Part model, mm, in its own coordinate system. A direction names the side the tool comes from. Round coordinates to 2 decimals unless told otherwise and drop trailing zeros. Loops run counter-clockwise (first coordinate to the right, second up) from the corner with the lowest first, then second, coordinate; pieces in that order, holes last. Notation, with made-up numbers: M -15,-7.5 L 0,-7.5 A16 ccw 0,8.5 Z; hole C 17,87 d9. An arc over 180 degrees is marked long. Write each question's results on one line, items separated by ' | '.
from build123d import *

# Parameters (mm, degrees)
SKETCH_W      = 13
SKETCH_H      = 10
PAD_DEPTH     = 1.6
SKETCH001_R   = 1.5
SKETCH001_W   = 0.65
SKETCH001_H   = 0.65
POCKET_DEPTH  = 5
SKETCH002_W   = 2.6
SKETCH002_H   = 2.6
PAD001_DEPTH  = 0.03
SKETCH003_W   = 2.1
SKETCH003_H   = 2.1
PAD002_DEPTH  = 0.9
FILLET_R      = 0.3
FILLET001_R   = 0.05
FILLET002_R   = 0.2
SKETCH004_W   = 1.1
SKETCH004_H   = 2
SKETCH004_W_2 = 1.5
SKETCH004_H_2 = 0.9
SKETCH004_H_3 = 0.75
SKETCH004_H_4 = 2.9
SKETCH004_W_3 = 3.2
SKETCH004_H_5 = 1.4
SKETCH004_W_4 = 0.8
SKETCH004_H_6 = 1.6
PAD003_DEPTH  = 0.27
SKETCH005_W   = 2.4
SKETCH005_H   = 2.4
PAD004_DEPTH  = 2.4
CHAMFER_SIZE  = 0.5
PAD005_DEPTH  = 2.4
SKETCH007_W   = 0.65
SKETCH007_H   = 0.65
PAD006_DEPTH  = 12


with BuildPart() as part:
    # Sketch (on XY_Plane of Origin) → Pad (new body)
    with BuildSketch(Plane.XY):
        with Locations((6.5, 5)):
            Rectangle(SKETCH_W, SKETCH_H)
    extrude(amount=PAD_DEPTH)

    # Sketch001 (on XY_Plane of Origin) → Pocket (cut)
    with BuildSketch(Plane.XY):
        with Locations((10.4, 7.6)):
            Circle(SKETCH001_R)
        with Locations((1.4, 8.6)):
            Rectangle(SKETCH001_W, SKETCH001_H)
        with Locations((1.4, 6.2)):
            Rectangle(SKETCH001_W, SKETCH001_H)
        with Locations((1.4, 3.8)):
            Rectangle(SKETCH001_W, SKETCH001_H)
        with Locations((1.4, 1.4)):
            Rectangle(SKETCH001_W, SKETCH001_H)
    extrude(amount=POCKET_DEPTH, mode=Mode.SUBTRACT)

    # Sketch002 (on Face5 of Pocket) → Pad001 (join)
    with BuildSketch(Plane.XY.offset(1.6)):
        with Locations((10.6, 2.7)):
            Rectangle(SKETCH002_W, SKETCH002_H)
    extrude(amount=PAD001_DEPTH)

    # Sketch003 (on Face28 of Pad001) → Pad002 (join)
    with BuildSketch(Plane.XY.offset(1.63)):
        with Locations((10.6, 2.7)):
            Rectangle(SKETCH003_W, SKETCH003_H)
    extrude(amount=PAD002_DEPTH)

    # Fillet
    fillet_edges = [part.edges().sort_by_distance(p)[0] for p in [
        (9.55, 1.65, 2.08),
        (9.55, 3.75, 2.08),
        (11.65, 1.65, 2.08),
        (11.65, 3.75, 2.08),
    ]]
    fillet(fillet_edges, radius=FILLET_R)

    # Fillet001
    fillet001_edges = [part.edges().sort_by_distance(p)[0] for p in [
        (9.637868, 1.737868, 1.63),
    ]]
    fillet(fillet001_edges, radius=FILLET001_R)

    # Fillet002
    fillet002_edges = [part.edges().sort_by_distance(p)[0] for p in [
        (10.6, 1.65, 2.53),
    ]]
    fillet(fillet002_edges, radius=FILLET002_R)

    # Sketch004 (on Face53 of Fillet002) → Pad003 (join)
    with BuildSketch(Plane(origin=(0, 0, 0), x_dir=(1, 0, 0), z_dir=(0, 0, -1))):
        with Locations((5.65, -2.1)):
            Rectangle(SKETCH004_W, SKETCH004_H)
        with Locations((8.7, -1.35)):
            Rectangle(SKETCH004_W_2, SKETCH004_H_2)
        with Locations((8.7, -2.95)):
            Rectangle(SKETCH004_W_2, SKETCH004_H_2)
        with Locations((8.7, -4.425)):
            Rectangle(SKETCH004_W_2, SKETCH004_H_3)
        with Locations((5.85, -7.65)):
            Rectangle(SKETCH004_W, SKETCH004_H_4)
        with Locations((4.8, -4.8)):
            Rectangle(SKETCH004_W_3, SKETCH004_H_5)
        with Locations((3.3, -8)):
            Rectangle(SKETCH004_W_4, SKETCH004_H_6)
    extrude(amount=PAD003_DEPTH)

    # Sketch005 (on Face53 of Pad003) → Pad004 (join)
    with BuildSketch(Plane(origin=(0, 0, 0), x_dir=(1, 0, 0), z_dir=(0, 0, -1))):
        with Locations((1.4, -1.4)):
            Rectangle(SKETCH005_W, SKETCH005_H)
        with Locations((1.4, -6.2)):
            Rectangle(SKETCH005_W, SKETCH005_H)
    extrude(amount=PAD004_DEPTH)

    # Chamfer
    chamfer_edges = [part.edges().sort_by_distance(p)[0] for p in [
        (2.6, 5, -1.2),
        (0.2, 5, -1.2),
        (2.6, 7.4, -1.2),
        (2.6, 2.6, -1.2),
        (2.6, 0.2, -1.2),
        (0.2, 0.2, -1.2),
        (0.2, 7.4, -1.2),
        (0.2, 2.6, -1.2),
    ]]
    chamfer(chamfer_edges, length=CHAMFER_SIZE)

    # Sketch006 (on Face1 of Chamfer) → Pad005 (join)
    with BuildSketch(Plane(origin=(0, 0, 0), x_dir=(1, 0, 0), z_dir=(0, 0, -1))):
        Polygon((0.7, -2.6), (2.1, -2.6), (2.6, -3.1), (2.6, -4.5), (2.1, -5), (0.7, -5), (0.2, -4.5), (0.2, -3.1), align=None)
        Polygon((0.7, -7.4), (2.1, -7.4), (2.6, -7.9), (2.6, -9.3), (2.1, -9.8), (0.7, -9.8), (0.2, -9.3), (0.2, -7.9), align=None)
    extrude(amount=PAD005_DEPTH)

    # Sketch007 (on Face61 of Pad005) → Pad006 (join)
    with BuildSketch(Plane.XY.offset(2.9)):
        with Locations((1.4, 8.6)):
            Rectangle(SKETCH007_W, SKETCH007_H)
        with Locations((1.4, 6.2)):
            Rectangle(SKETCH007_W, SKETCH007_H)
        with Locations((1.4, 3.8)):
            Rectangle(SKETCH007_W, SKETCH007_H)
        with Locations((1.4, 1.4)):
            Rectangle(SKETCH007_W, SKETCH007_H)
    extrude(amount=-PAD006_DEPTH)


solid = part.part
Item 1: Band-saw the part on C-C on z = -6.75. Give the cut face in (x, y) (3 decimals).
Filled sheet:
outline: M 1.075,1.075 L 1.725,1.075 L 1.725,1.725 L 1.075,1.725 Z; M 1.075,3.475 L 1.725,3.475 L 1.725,4.125 L 1.075,4.125 Z; M 1.075,5.875 L 1.725,5.875 L 1.725,6.525 L 1.075,6.525 Z; M 1.075,8.275 L 1.725,8.275 L 1.725,8.925 L 1.075,8.925 Z
Item 2: Band-saw the part on D-D on x = 7. Give the cut face in (y, z), and give its area (3 significant figures).
Filled sheet:
outline: M 0,0 L 10,0 L 10,1.6 L 0,1.6 Z | area: 16.0 mm^2
Item 3: Which spindle directions (+Z, -Z, +X, -X, +Y, -Y) get a long thin tool onto all of the face, cutting with end or side? Do faces 4 (the flat face through (6, 0, 1)), 5 (the flat face through (5, 5, -0.27)), 6 (the flat face through (1, 0.2, -1)), 7 (the flat face through (0, 5, 1)), 8 (the flat face through (0.2, 4, -1)). Say none if no direction does.
Filled sheet:
face 4: +Z, -Z, +X, -X, -Y | face 5: -Z, +X, +Y, -Y | face 6: -Z, +X, -X, -Y | face 7: +Z, -Z, -X, +Y, -Y | face 8: -Z, -X, +Y, -Y
Item 4: Drop flat-ended pins along their axis: P1, Ø0.5, axis at x = 10.5, y = 3, coming from the +Z side; P2, Ø2, axis at x = 2, z = -6, coming from the -Y side (3 decimals); P3, Ø1.5, axis at y = 4, z = -3, coming from the +X side; P4, Ø1, axis at x = 11, z = 0, coming from the -Y side. Give the stop position or say it passes through.
Filled sheet:
P1: z = 2.53 | P2: y = 1.075 | P3: x = 2.6 | P4: y = 0
Item 5: Wall check: L1, parallel to Y at x = 10.4, z = 0.5; L2, parallel to Z at x = 9.75, y = 2; L3, parallel to Z at x = 7.75, y = 4. Give the ranges that are in metal, low to high.
Filled sheet:
L1: 0 to 6.1, 9.1 to 10 | L2: 0 to 2.53 | L3: 0 to 1.6
Item 6: Band-saw the part on A-A on y = 7.6. Give the cut face in (x, z), and give its area (3 significant figures).
Filled sheet:
outline: M 0,0 L 0.5,0 L 0.5,-2.4 L 2.3,-2.4 L 2.3,0 L 2.9,0 L 2.9,-0.27 L 3.7,-0.27 L 3.7,0 L 5.3,0 L 5.3,-0.27 L 6.4,-0.27 L 6.4,0 L 8.9,0 L 8.9,1.6 L 0,1.6 Z; M 11.9,0 L 13,0 L 13,1.6 L 11.9,1.6 Z | area: 20.8 mm^2
Item 7: Two-plate mould, pull along Y, no slides. Class faces 1 (the flat face through (0.2, 9, -1)), 2 (the flat face through (6, 10, 1)), 3 (the cylindrical face through (9.29, 8.61, 0.79)): +Y half, -Y half, draft (parallel to the pull), parting line (faces both ways), or undercut.
Filled sheet:
face 1: draft | face 2: +Y half | face 3: undercut
